Read the model definition and answer for the solid it produces. Units are mm, in the model's axes. Face numbers are marked on the shaded views. A direction names the side the tool comes from. Coordinates: 2 decimals unless noted, no trailing zeros. Write each loop counter-clockwise with the first axis right and the second up, starting at its lowest first coordinate (ties: lowest second). Pieces come first, ordered by that corner, then holes.
(1) The part is cut by section D-D, the plane z = 11. Determine the outline of the cut face in (x, y), and give its area (3 significant figures).
(2) The part is cut by section A-A, the plane x = 1. Determine the outline of the cut face in (y, z), and give its area (3 significant figures).
(3) The part is cut by section B-B, the plane x = -14.5. Determine the outline of the cut face in (y, z).
(4) Given pin 1 (3.5 mm diameter, centred on x = 1.5, y = -15, fed in from +Z); pin 2 (1.5 mm diameter, centred on x = -5.5, z = 18.5, fed in from +Y); pin 3 (8 mm diameter, centred on y = -14, z = 22.5, fed in from -X); pin 4 (4.5 mm diameter, centred on x = -14.5, y = 0, fed in from -Z), each flat-ended and moving along its own axis, determine where each tip first touches the part or whether it passes through.
(5) Straight lines are drawn through the part: line 1 along X through (y, z) = (0, 52.15); line 2 along X through (y, z) = (0, 50.2). For each, find the intervals that lie inside material, in ascending order.
(6) Which of the six approach directions +Z, -Z, +X, -X, +Y, -Y give full straight-line access (tool end or side, diameter ignored) to the marked faces 1, 2 and 3?
(7) The part is cut by section C-C, the plane y = -13.5. Determine the outline of the cut face in (x, z), and give its area (3 significant figures).
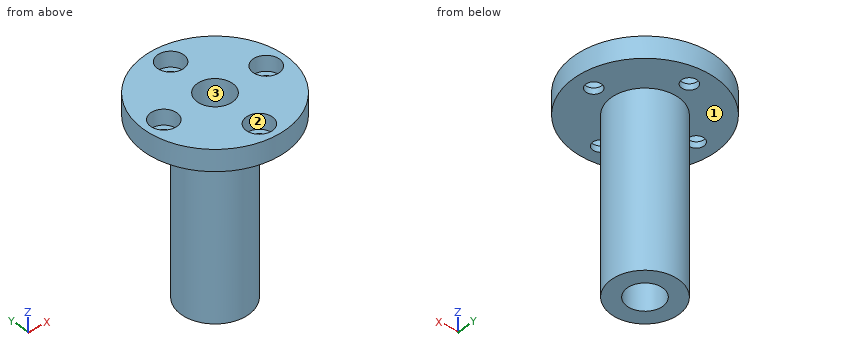
Autodesk Inventor part; units mm, degrees
ref_plane "YZ Plane" through (0, 0, 0) normal (1, 0, 0) x (0, 1, 0)
ref_plane "XZ Plane" through (0, 0, 0) normal (0, 1, 0) x (-1, 0, 0)
ref_plane "XY Plane" through (0, 0, 0) normal (0, 0, 1) x (1, 0, 0)
sketch "スケッチ2" plane through (0, 0, 0) normal (1, 0, 0) x (0, 1, 0)
  line L0 (5, 0) -> (9.5, 0)
  line L1 (9.5, 0) -> (9.5, 49)
  line L2 (9.5, 49) -> (20, 49)
  line L3 (20, 49) -> (20, 55)
  line L4 (20, 55) -> (5, 55)
  line L5 (5, 0) -> (5, 55)
  line L6 (0, -11) -> (0, 66)
  point P0 (0, 0)
  point P1 (0, 55)
  dimension "d0" = 9.5
  dimension "d1" = 55
  dimension "d2" = 6
  dimension "d3" = 20
  dimension "d4" = 5
revolve "回転1" add sketch "スケッチ2" angle 360 about axis through (0, 0, -10) along (0, 0, 1)
sketch "スケッチ3" plane through (0, 0, 55) normal (0, 0, 1) x (1, 0, 0)
  circle A0 centre (0, 14.5) radius 3.7
  point P0 (0, 0)
  dimension "d6" = 14.5
  dimension "d7" = 7.4
extrude "押し出し1" cut sketch "スケッチ3" against normal blind 4.3
sketch "スケッチ4" plane through (0, 14.5, 50.7) normal (0, 0, 1) x (1, 0, 0)
  circle A0 centre (0, 0) radius 2.2
  circle A1 centre (0, 0) radius 3.7
  point P0 (0, -14.5)
  dimension "d10" = 4.4
extrude "押し出し2" cut sketch "スケッチ4" against normal through all contours A0
pattern_circular "円形状パターン1" count 4 over 360 about axis through (0, 0, -10) along (0, 0, 1) of "押し出し1", "押し出し2"
equation "\"d1\" = L"
equation "\"d2\" = t"
equation "\"D\" = 19"
equation "\"L\" = 55"
equation "\"t\" = 6"
equation "\"PCD\" = 29"
properties part number "NB_SMF10WW"
Computed:
1. outline: circle Ø19 at (0, 0); hole circle Ø10 at (0, 0)
1. area: 205 mm2
2. outline: (-19.97, 49) - (-16.46, 49) - (-16.46, 50.7) - (-18.06, 50.7) - (-18.06, 55) - (-19.97, 55) - close; (-12.54, 49) - (-9.45, 49) - (-9.45, 0) - (-4.9, 0) - (-4.9, 55) - (-10.94, 55) - (-10.94, 50.7) - (-12.54, 50.7) - close; (4.9, 0) - (9.45, 0) - (9.45, 49) - (12.54, 49) - (12.54, 50.7) - (10.94, 50.7) - (10.94, 55) - (4.9, 55) - close; (16.46, 49) - (19.97, 49) - (19.97, 55) - (18.06, 55) - (18.06, 50.7) - (16.46, 50.7) - close
2. area: 552 mm2
3. outline: (-13.77, 49) - (-2.2, 49) - (-2.2, 50.7) - (-3.7, 50.7) - (-3.7, 55) - (-13.77, 55) - close; (2.2, 49) - (13.77, 49) - (13.77, 55) - (3.7, 55) - (3.7, 50.7) - (2.2, 50.7) - close
4. pin 1: stops at z = 50.7
4. pin 2: stops at y = 8.23
4. pin 3: passes through
4. pin 4: stops at z = 49
5. line 1: x = -20 to -18.2, -10.8 to -5, 5 to 10.8, 18.2 to 20
5. line 2: x = -20 to -16.7, -12.3 to -5, 5 to 12.3, 16.7 to 20
6. face 1: -Z
6. face 2: +Z
6. face 3: +Z, -Z
7. outline: (-14.76, 49) - (-1.96, 49) - (-1.96, 50.7) - (-3.56, 50.7) - (-3.56, 55) - (-14.76, 55) - close; (1.96, 49) - (14.76, 49) - (14.76, 55) - (3.56, 55) - (3.56, 50.7) - (1.96, 50.7) - close
7. area: 140 mm2
